from build123d import *

# Parameters (mm, degrees)
F0_R      = 50.5719181769
F1_DEPTH  = 152.4
F2_W      = 45.1020896435
F2_H      = 153.3471494913
F3_DEPTH  = 25.4
F4_W      = 45.3240573406
F4_H      = 153.6485850811
F5_DEPTH  = 25.4
F7_DEPTH  = 25.4
F8_R      = 14.8077748838
F7_FACE_W = 46.2437570095
F7_FACE_H = 148.4715342522
F9_DEPTH  = 12.7
F10_R     = 14.8077748838
F11_DEPTH = 25.4
F12_R     = 14.0159592486
F13_DEPTH = 25.4
F14_R     = 12.7922507372
F15_DEPTH = 25.4
F16_R     = 19.6873563426
F17_DEPTH = 177.8
F18_R     = 24.1990782375
F19_DEPTH = 101.6
F20_DEPTH = 25.4
F21_DEPTH = 203.2


with BuildPart() as f1:
    # F0 (on Right) → F1 (new body)
    with BuildSketch(Plane.YZ):
        Circle(F0_R)
    extrude(amount=F1_DEPTH)

    # F2 (on Right) → F3 (join)
    with BuildSketch(Plane.YZ):
        with Locations((0, 32.645329833)):
            Rectangle(F2_W, F2_H)
    extrude(amount=F3_DEPTH)

    # F4 (on Right) → F5 (join)
    with BuildSketch(Plane.YZ):
        with Locations((0, 31.9696366787)):
            Rectangle(F4_W, F4_H)
    extrude(amount=F5_DEPTH)

    # F6 (on face) → F7 (join)
    with BuildSketch(Plane.YZ.offset(152.4)):
        with BuildLine():
            ThreePointArc((23.1218785048, 44.9766344061), (0, 50.5719181769), (-23.1218785048, 44.9766344061))
            Line((-23.1218785048, 44.9766344061), (-23.1218785048, -39.3963605165))
            Line((-23.1218785048, -39.3963605165), (23.1218785048, -39.3963605165))
            Line((23.1218785048, -39.3963605165), (23.1218785048, 44.9766344061))
        make_face()
        with BuildLine():
            Line((23.1218785048, 109.0751737356), (-23.1218785048, 109.0751737356))
            Line((-23.1218785048, 109.0751737356), (-23.1218785048, 44.9766344061))
            ThreePointArc((-23.1218785048, 44.9766344061), (0, 50.5719181769), (23.1218785048, 44.9766344061))
            Line((23.1218785048, 44.9766344061), (23.1218785048, 109.0751737356))
        make_face()
    extrude(amount=F7_DEPTH)

    # F8 (on Right) + F7_face (on face) → F9 (cut, symmetric)
    with BuildSketch(Plane.YZ):
        with Locations((0, 81.6606134176)):
            Circle(F8_R)
    with BuildSketch(Plane(origin=(177.8, 0, 34.8394066095), x_dir=(0, 1, 0), z_dir=(1, 0, 0))):
        Rectangle(F7_FACE_W, F7_FACE_H)
    extrude(amount=F9_DEPTH, both=True, mode=Mode.SUBTRACT)

    # F10 (on face) → F11 (cut)
    with BuildSketch(Plane(origin=(12.7, 0, 0), x_dir=(0, -1, 0), z_dir=(-1, 0, 0))):
        with Locations((0, 81.6606134176)):
            Circle(F10_R)
    extrude(amount=-F11_DEPTH, mode=Mode.SUBTRACT)

    # F12 (on Right) → F13 (cut)
    with BuildSketch(Plane.YZ):
        with Locations((-7.2993179783, 64.5171701908)):
            Circle(F12_R)
    extrude(amount=-F13_DEPTH, mode=Mode.SUBTRACT)

    # F14 (on face) → F15 (cut)
    with BuildSketch(Plane(origin=(152.4, 0, 0), x_dir=(0, -1, 0), z_dir=(-1, 0, 0))):
        with Locations((0, 90.3855785728)):
            Circle(F14_R)
    extrude(amount=-F15_DEPTH, mode=Mode.SUBTRACT)

    # F16 (on Right) → F17 (cut)
    with BuildSketch(Plane.YZ):
        Circle(F16_R)
    extrude(amount=-F17_DEPTH, mode=Mode.SUBTRACT)

    # F18 (on Right) → F19 (cut, symmetric)
    with BuildSketch(Plane.YZ):
        Circle(F18_R)
    extrude(amount=F19_DEPTH, both=True, mode=Mode.SUBTRACT)

    # F20 (cut): a face of the model
    f20_faces = [f1.faces().sort_by_distance(p)[0] for p in [
        (101.6, 0, 0),
    ]]
    extrude(f20_faces, amount=-F20_DEPTH, mode=Mode.SUBTRACT)

    # F21 (cut): a face of the model
    f21_faces = [f1.faces().sort_by_distance(p)[0] for p in [
        (127, 0, 0),
    ]]
    extrude(f21_faces, amount=-F21_DEPTH, mode=Mode.SUBTRACT)


solid = f1.part
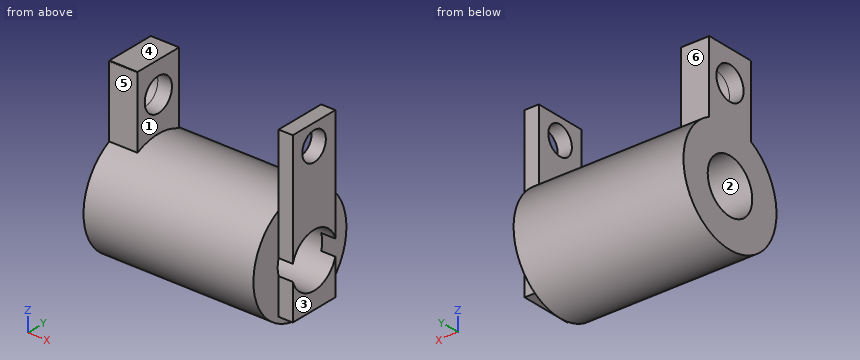
Verification items for the finished model (mm, model axes). Face numbers are marked on the shaded views. A direction names the side the tool comes from. Coordinates: 2 decimals unless noted, no trailing zeros. Write each loop counter-clockwise with the first axis right and the second up, starting at its lowest first coordinate (ties: lowest second). Pieces come first, ordered by that corner, then holes. Notation, with made-up numbers: (7.5, 20.25) - (24.5, 20.25) arc R26 ccw to (24.5, 42.25) - close; hole circle Ø10 at (-17, 66.25). An arc over 180 degrees is marked (long way). Answer as a JSON object with one key per item and string values.
(1) Cross-section at A-A on z = 0. Record the cut outline in (x, y).
Report:
{"outline": "(0, -50.57) - (152.4, -50.57) - (152.4, -24.2) - (0, -24.2) - close; (0, 24.2) - (152.4, 24.2) - (152.4, 50.57) - (0, 50.57) - close"}
(2) Thickness scan on line 1 along Z through (x, y) = (20.5, 0); line 2 along Z through (x, y) = (160.75, 0); line 3 along X through (y, z) = (-40.5, -3). Record the ranges inside material, lowest first.
Report:
{"line 1": "-50.57 to -24.2, 24.2 to 66.85, 96.47 to 109.32", "line 2": "-39.4 to -24.2, 24.2 to 77.59, 103.18 to 109.08", "line 3": "0 to 152.4"}
(3) Gauge pin test, flat ends, axial feed: pin 1 Ø4 at (x, z) = (158.5, -22.5) entering from -Y; pin 2 Ø14 at (x, y) = (161.5, -0.5) entering from -Z; pin 3 Ø5 at (x, z) = (100.5, -9.5) entering from +Y. Record the tip position at first contact, or that the pin passes through.
Report:
{"pin 1": "y = -23.12", "pin 2": "z = -39.4", "pin 3": "y = 50.09"}
(4) Mould release check, pull along X, two halves, no side actions. Record for the marked faces 1, 2 and 3: pulls with the +X half, pulls with the -X half, needs draft (parallel to the pull), parting line crosses it, or undercut.
Report:
{"face 1": "undercut", "face 2": "needs draft", "face 3": "pulls with the +X half"}
(5) Cross-section at B-B on y = 0. Record the cut outline in (x, z), plus the area to 3 significant figures.
Report:
{"outline": "(0, -50.57) - (152.4, -50.57) - (152.4, -39.4) - (165.1, -39.4) - (165.1, -24.2) - (0, -24.2) - close; (0, 24.2) - (165.1, 24.2) - (165.1, 77.59) - (152.4, 77.59) - (152.4, 50.57) - (25.4, 50.57) - (25.4, 66.85) - (0, 66.85) - close; (0, 96.47) - (25.4, 96.47) - (25.4, 109.32) - (0, 109.32) - close; (152.4, 103.18) - (165.1, 103.18) - (165.1, 109.08) - (152.4, 109.08) - close", "area": "9,720 mm^2"}
(6) Tool access check on the marked faces 4, 5 and 6. Record the directions out of +Z, -Z, +X, -X, +Y, -Y that give a thin tool (end or side, any length) a straight path to the whole face; none if there is none.
Report:
{"face 4": "+Z, +X, -X, +Y, -Y", "face 5": "+Z, -X, -Y", "face 6": "+Z, -X, +Y"}
(7) Cross-section at C-C on z = 92.5. Record the cut outline in (x, y).
Report:
{"outline": "(0, -22.66) - (25.4, -22.66) - (25.4, -10.09) - (0, -10.09) - close; (0, 10.09) - (25.4, 10.09) - (25.4, 22.66) - (0, 22.66) - close; (152.4, -23.12) - (165.1, -23.12) - (165.1, -12.62) - (152.4, -12.62) - close; (152.4, 12.62) - (165.1, 12.62) - (165.1, 23.12) - (152.4, 23.12) - close"}
(8) Cross-section at D-D on x = 20. Record the cut outline in (y, z), plus the area to 3 significant figures.
Report:
{"outline": "(-22.66, 45.21) arc R50.57 ccw (long way) to (22.66, 45.21) - (22.66, 108.79) - (22.55, 108.79) - (22.55, 109.32) - (-22.55, 109.32) - (-22.55, 108.79) - (-22.66, 108.79) - close; hole circle Ø48.4 at (0, 0); hole circle Ø29.62 at (0, 81.66)", "area": "8,250 mm^2"}
